Here's how the part is built. I have some questions about the finished solid (model axes, mm). A direction names the side the tool comes from. Coordinates: 2 decimals unless noted, no trailing zeros. Write each loop counter-clockwise with the first axis right and the second up, starting at its lowest first coordinate (ties: lowest second). Pieces come first, ordered by that corner, then holes.
```python
from build123d import *

# Parameters (mm, degrees)
SKETCH1_W           = 78
SKETCH1_H           = 12
BOSS_EXTRUDE1_DEPTH = 35
SKETCH1_4_R         = 4
CUT_EXTRUDE1_DEPTH  = 27
SKETCH1_5_R         = 1.6
CUT_EXTRUDE2_DEPTH  = 35
SKETCH1_6_R         = 1.621
CUT_EXTRUDE3_DEPTH  = 12


with BuildPart() as part:
    # Sketch1 → Boss-Extrude1 (new body)
    with BuildSketch(Plane(origin=(0, 0, 0), x_dir=(0, 0, -1), z_dir=(1, 0, 0))):
        Rectangle(SKETCH1_W, SKETCH1_H)
    extrude(amount=BOSS_EXTRUDE1_DEPTH)

    # Sketch1<4> → Cut-Extrude1 (cut)
    with BuildSketch(Plane(origin=(0, 0, 0), x_dir=(0, 0, -1), z_dir=(1, 0, 0))):
        with Locations((-20, 0)):
            Circle(SKETCH1_4_R)
        with Locations((20, 0)):
            Circle(SKETCH1_4_R)
    extrude(amount=CUT_EXTRUDE1_DEPTH, mode=Mode.SUBTRACT)

    # Sketch1<5> → Cut-Extrude2 (cut)
    with BuildSketch(Plane(origin=(0, 0, 0), x_dir=(0, 0, -1), z_dir=(1, 0, 0))):
        with Locations((-20, 0)):
            Circle(SKETCH1_5_R)
        with Locations((20, 0)):
            Circle(SKETCH1_5_R)
    extrude(amount=CUT_EXTRUDE2_DEPTH, mode=Mode.SUBTRACT)

    # Sketch1<6> → Cut-Extrude3 (cut)
    with BuildSketch(Plane(origin=(0, 0, 0), x_dir=(0, 0, -1), z_dir=(1, 0, 0))):
        with Locations((-34, 0)):
            Circle(SKETCH1_6_R)
        with Locations((34, 0)):
            Circle(SKETCH1_6_R)
    extrude(amount=CUT_EXTRUDE3_DEPTH, mode=Mode.SUBTRACT)


solid = part.part
```
1) On a 3-axis mill with a long thin cutter (end or side, diameter ignored), from which of +Z, -Z, +X, -X, +Y, -Y can I reach the whole of each face in a straight line? I mean faces 4 (the face through (12, 0, 34)), 5 (the face through (17, -6, 1)). Say none if no direction works.
Values follow:
face 4: -X
face 5: +Z, -Z, +X, -X, -Y
2) Imagine slicing it at B-B on y = 0. Please give me the cut outline in (x, z).
Values follow:
outline: (0, -39) - (35, -39) - (35, -21.6) - (27, -21.6) - (27, -24) - (0, -24) - (0, -32.38) - (12, -32.38) - (12, -35.62) - (0, -35.62) - close; (0, -16) - (27, -16) - (27, -18.4) - (35, -18.4) - (35, 18.4) - (27, 18.4) - (27, 16) - (0, 16) - close; (0, 24) - (27, 24) - (27, 21.6) - (35, 21.6) - (35, 39) - (0, 39) - (0, 35.62) - (12, 35.62) - (12, 32.38) - (0, 32.38) - close
3) Will these pins go through, and if not, where does the flat tip stop? pin 1 (1 mm diameter, centred on y = 4.5, z = 1.5, fed in from -X); pin 2 (4 mm diameter, centred on y = 1, z = 19.5, fed in from -X); pin 3 (3 mm diameter, centred on y = 0, z = 20, fed in from +X); pin 4 (1 mm diameter, centred on y = -0.5, z = 34, fed in from -X).
Values follow:
pin 1: stops at x = 0
pin 2: stops at x = 27
pin 3: passes through
pin 4: stops at x = 12
4) I need wall thicknesses on probe 1 along Z at (x, y) = (29, 0); probe 2 along Z at (x, y) = (20, 0.25); probe 3 along Y at (x, z) = (32.5, 20). Which ranges of each line are inside material? Lowest first, please.
Values follow:
probe 1: z = -39 to -21.6, -18.4 to 18.4, 21.6 to 39
probe 2: z = -39 to -23.99, -16.01 to 16.01, 23.99 to 39
probe 3: y = -6 to -1.6, 1.6 to 6
5) Imagine slicing it at A-A on z = 20. Please give me the cut outline in (x, y), then the cut area to 3 significant figures.
Values follow:
outline: (0, -6) - (35, -6) - (35, -1.6) - (27, -1.6) - (27, -4) - (0, -4) - close; (0, 4) - (27, 4) - (27, 1.6) - (35, 1.6) - (35, 6) - (0, 6) - close
area: 178 mm2
6) Imagine slicing it at D-D on x = 21.5. Please give me the cut outline in (y, z), then the cut area to 3 significant figures.
Values follow:
outline: (-6, -39) - (6, -39) - (6, 39) - (-6, 39) - close; hole circle Ø8 at (0, -20); hole circle Ø8 at (0, 20)
area: 835 mm2
7) Imagine slicing it at C-C on z = -34. Please give me the cut outline in (x, y).
Values follow:
outline: (0, -6) - (35, -6) - (35, 6) - (0, 6) - (0, 1.62) - (12, 1.62) - (12, -1.62) - (0, -1.62) - close
8) We'd pull the mould along Y, two halves only. Please class faces 1 (the face through (17, 6, 1)), 2 (the face through (30.94, 1.08, 21.18)), 3 (the face through (35, 0, 1)): pulls with the +Y half, pulls with the -Y half, needs draft (parallel to the pull), parting line crosses it, or undercut.
Values follow:
face 1: pulls with the +Y half
face 2: undercut
face 3: needs draft
